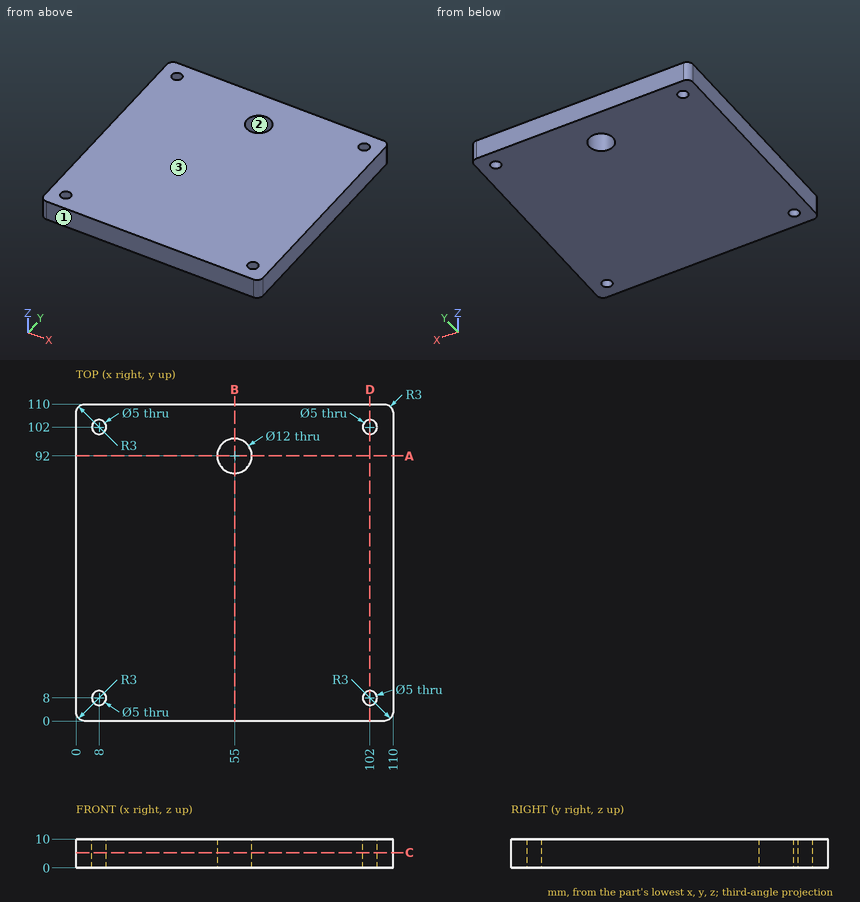
Geometry: see drawing. Coordinates: mm, zero at the bounding-box minimum. Round coordinates to 2 decimals unless told otherwise and drop trailing zeros. Loops run counter-clockwise (first coordinate to the right, second up) from the corner with the lowest first, then second, coordinate; pieces in that order, holes last. Notation, with made-up numbers: (88.25, 1) - (104.25, 1) arc R33 ccw to (104.25, 30) - close; hole circle Ø4 at (57.25, -2). An arc over 180 degrees is marked (long way). One line per item, written item: value. Start each with the question number.
(1) Section B-B, the plane x = 55. Return loops of the section in (y, z), plus the area to 3 significant figures.
(2) Section A-A, the plane y = 92. Return loops of the section in (x, z), plus the area to 3 significant figures.
(3) Section D-D, the plane x = 102. Return loops of the section in (y, z), plus the area to 3 significant figures.
(4) Draft query along Y for the marked faces 1, 2 and 3. Return one class per face: +Y half, -Y half, draft (parallel to the pull), parting line (faces both ways), or undercut.
(5) Ray query, line 1 (Y direction, x = 8, z = 4.25); line 2 (Y direction, x = 55, z = 5.5). Return the intervals inside material, ascending. Write a range as [from, to].
(6) Section C-C, the plane z = 5.25. Return loops of the section in (x, y), plus the area to 3 significant figures.
(7) Contact query for a flat-ended pin moving along its axis: P1, Ø3, axis at x = 8, y = 102, coming from the -Z side. Output: stop coordinate, or through.
Results below:
1. outline: (0, 0) - (86, 0) - (86, 10) - (0, 10) - close; (98, 0) - (110, 0) - (110, 10) - (98, 10) - close
1. area: 980 mm^2
2. outline: (0, 0) - (49, 0) - (49, 10) - (0, 10) - close; (61, 0) - (110, 0) - (110, 10) - (61, 10) - close
2. area: 980 mm^2
3. outline: (0, 0) - (5.5, 0) - (5.5, 10) - (0, 10) - close; (10.5, 0) - (99.5, 0) - (99.5, 10) - (10.5, 10) - close; (104.5, 0) - (110, 0) - (110, 10) - (104.5, 10) - close
3. area: 1,000 mm^2
4. face 1: -Y half
4. face 2: undercut
4. face 3: draft
5. line 1: [0, 5.5], [10.5, 99.5], [104.5, 110]
5. line 2: [0, 86], [98, 110]
6. outline: (0, 3) arc R3 ccw to (3, 0) - (107, 0) arc R3 ccw to (110, 3) - (110, 107) arc R3 ccw to (107, 110) - (3, 110) arc R3 ccw to (0, 107) - close; hole circle Ø5 at (8, 8); hole circle Ø5 at (8, 102); hole circle Ø12 at (55, 92); hole circle Ø5 at (102, 8); hole circle Ø5 at (102, 102)
6. area: 11,900 mm^2
7. P1: through
